Here's how the part is built. I have some questions about the finished solid (model axes, mm). Face numbers are marked on the shaded views. A direction names the side the tool comes from. Give positions to 0.01 mm unless a question says otherwise; leave off trailing zeros. Write each loop counter-clockwise with the first axis right and the second up, starting at its lowest first coordinate (ties: lowest second). Pieces come first, ordered by that corner, then holes. Notation, with made-up numbers: (59, -4) -> (94, -4) arc R15 ccw to (94, 0) -> close; hole circle Ø2 at (40.5, 33.25). An arc over 180 degrees is marked (long way). Return JSON: item names as keys, results as strings.
from build123d import *

# Parameters (mm, degrees)
SKETCH_1_W      = 25.1
SKETCH_1_H      = 19
EXTRUDE_1_DEPTH = 0.8
SKETCH_2_W      = 12.4
SKETCH_2_H      = 17
EXTRUDE_2_DEPTH = 3.75
EXTRUDE_3_DEPTH = 0.1


with BuildPart() as part:
    # Эскиз1 → Бобышка-Вытянуть1 (new body)
    with BuildSketch(Plane.XY):
        Rectangle(SKETCH_1_W, SKETCH_1_H)
    extrude(amount=EXTRUDE_1_DEPTH)

    # Эскиз2 → Бобышка-Вытянуть2 (add)
    with BuildSketch(Plane.XY.offset(0.8)):
        with Locations((-6.35, 0)):
            Rectangle(SKETCH_2_W, SKETCH_2_H)
        with Locations((6.35, 0)):
            Rectangle(SKETCH_2_W, SKETCH_2_H)
    extrude(amount=EXTRUDE_2_DEPTH)

    # Эскиз3 → Бобышка-Вытянуть3 (add)
    with BuildSketch(Plane.XY.offset(4.55)):
        Polygon((-2.02468415, 6.47520488), (-2.557441739, 7.110113629), (-7.634747282, 7.110113629), (-8.413649878, 6.456542649), (-7.703502871, 5.610259577), (-3.055232199, 5.610259577), align=None)
        Polygon((-1.29882158, 5.610259577), (-2.115441527, 0.979668914), (-3.03146241, 0.211374323), (-3.644937808, 0.942733655), (-2.862323662, 5.380419467), (-1.831775613, 6.245561214), align=None)
        Polygon((-7.933342981, 5.41735104), (-8.715781578, 0.979668914), (-9.631802461, 0.211374323), (-10.245102311, 0.942933785), (-9.422392583, 5.610259577), (-8.643686432, 6.263830557), align=None)
        Polygon((-8.523069486, 0.750025248), (-3.874798814, 0.750025248), (-3.260537626, 0), (-4.176367833, -0.749828804), (-8.824808297, -0.749828804), (-9.438886615, 0), align=None)
        Polygon((-3.984111693, -0.979995723), (-3.06780465, -0.211374323), (-2.454394697, -0.942560314), (-3.277521077, -5.609847275), (-4.056117123, -6.263437667), (-4.766565605, -5.416832984), align=None)
        Polygon((-9.054648407, -0.942737341), (-9.668341145, -0.211177879), (-10.584362029, -0.979472469), (-11.400981975, -5.609866688), (-10.868224387, -6.244775436), (-9.837186085, -5.37955138), align=None)
        Polygon((-4.996497129, -5.609866688), (-9.644374912, -5.609866688), (-10.674989606, -6.475066276), (-10.142165372, -7.110113629), (-5.064859829, -7.110113629), (-4.286153678, -6.456346204), align=None)
        Polygon((10.67560373, 6.47520488), (10.142846141, 7.110113629), (5.065540598, 7.110113629), (4.286638002, 6.456542649), (4.996785009, 5.610259577), (9.64505568, 5.610259577), align=None)
        Polygon((11.4014663, 5.610259577), (10.584846353, 0.979668914), (9.66882547, 0.211374323), (9.055350072, 0.942733655), (9.837964217, 5.380419467), (10.868512267, 6.245561214), align=None)
        Polygon((4.766944899, 5.41735104), (3.984506302, 0.979668914), (3.068485419, 0.211374323), (2.455185569, 0.942933785), (3.277895297, 5.610259577), (4.056601448, 6.263830557), align=None)
        Polygon((4.177218394, 0.750025248), (8.825489066, 0.750025248), (9.439750254, 0), (8.523920047, -0.749828804), (3.875479583, -0.749828804), (3.261401265, 0), align=None)
        Polygon((8.716176187, -0.979995723), (9.63248323, -0.211374323), (10.245893183, -0.942560314), (9.422766803, -5.609847275), (8.644170756, -6.263437667), (7.933722275, -5.416832984), align=None)
        Polygon((3.645639473, -0.942737341), (3.031946734, -0.211177879), (2.115925851, -0.979472469), (1.299305904, -5.609866688), (1.832063493, -6.244775436), (2.863101795, -5.37955138), align=None)
        Polygon((7.70379075, -5.609866688), (3.055912968, -5.609866688), (2.025298274, -6.475066276), (2.558122507, -7.110113629), (7.635428051, -7.110113629), (8.414134202, -6.456346204), align=None)
    extrude(amount=EXTRUDE_3_DEPTH)


solid = part.part
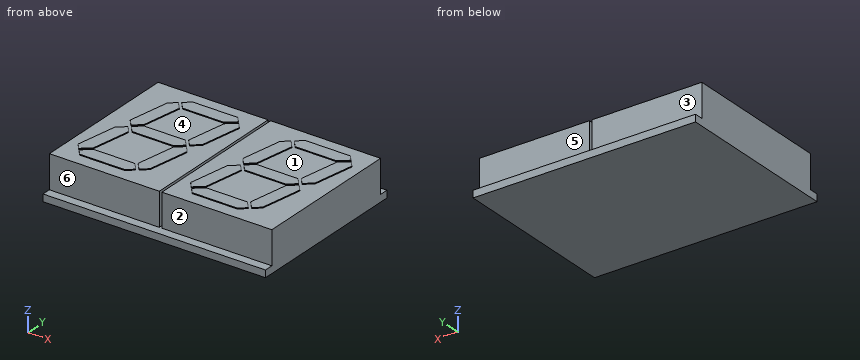
1. If I drill on line 1 (X direction, y = -7.5, z = 4.25); line 2 (Y direction, x = 2.75, z = 3.55); line 3 (Z direction, x = -4.75, y = -3.25), over which ranges is the centre line in solid material (lowest first)? Write a range as [from, to].
Taken from the geometry:
{"line 1": "x = [-12.55, -0.15], [0.15, 12.55]", "line 2": "y = [-8.5, 8.5]", "line 3": "z = [0, 4.55]"}
2. Suppose I cut it at A-A, the plane x = 1. List the corners of the cut face in (y, z) for me, and give its area (4 significant figures).
Taken from the geometry:
{"outline": "(-9.5, 0) -> (9.5, 0) -> (9.5, 0.8) -> (8.5, 0.8) -> (8.5, 4.55) -> (-8.5, 4.55) -> (-8.5, 0.8) -> (-9.5, 0.8) -> close", "area": "78.95 mm²"}
3. If we mould it in two halves opening along Y, with no side actions, what happens to the marked faces 1, 2 and 3? For each: released by +Y, released by -Y, zero draft, split by the parting line, or undercut.
Taken from the geometry:
{"face 1": "undercut", "face 2": "released by -Y", "face 3": "released by +Y"}
4. Suppose I cut it at D-D, the plane y = 4. List the corners of the cut face in (x, z) for me.
Taken from the geometry:
{"outline": "(-12.55, 0) -> (12.55, 0) -> (12.55, 4.55) -> (11.12, 4.55) -> (11.12, 4.65) -> (9.59, 4.65) -> (9.59, 4.55) -> (4.52, 4.55) -> (4.52, 4.65) -> (2.99, 4.65) -> (2.99, 4.55) -> (0.15, 4.55) -> (0.15, 0.8) -> (-0.15, 0.8) -> (-0.15, 4.55) -> (-1.58, 4.55) -> (-1.58, 4.65) -> (-3.11, 4.65) -> (-3.11, 4.55) -> (-8.18, 4.55) -> (-8.18, 4.65) -> (-9.71, 4.65) -> (-9.71, 4.55) -> (-12.55, 4.55) -> close"}
5. Suppose I cut it at C-C, the plane y = 7.75. List the corners of the cut face in (x, z) for me, and give its area (3 significant figures).
Taken from the geometry:
{"outline": "(-12.55, 0) -> (12.55, 0) -> (12.55, 4.55) -> (0.15, 4.55) -> (0.15, 0.8) -> (-0.15, 0.8) -> (-0.15, 4.55) -> (-12.55, 4.55) -> close", "area": "113 mm²"}
6. For pin 1 Ø1.1 at (x, z) = (4, 3) entering from +Y; pin 2 Ø1.5 at (x, y) = (-2, -4) entering from +Z; pin 3 Ø1.9 at (x, z) = (4.5, 3.5) entering from -Y, each with a flat end and sliding along its axis, tell me the tip position at first contact or that it passes through.
Taken from the geometry:
{"pin 1": "stops at y = 8.5", "pin 2": "stops at z = 4.55", "pin 3": "stops at y = -8.5"}
7. Suppose I cut it at B-B, the plane z = 2.95. List the corners of the cut face in (x, y) for me, and give its area (3 significant figures).
Taken from the geometry:
{"outline": "(-12.55, -8.5) -> (-0.15, -8.5) -> (-0.15, 8.5) -> (-12.55, 8.5) -> close; (0.15, -8.5) -> (12.55, -8.5) -> (12.55, 8.5) -> (0.15, 8.5) -> close", "area": "422 mm²"}
8. Which directions (+Z, -Z, +X, -X, +Y, -Y) give clear straight access to the entire face, cutting with the end or side of a thin tool? Please do the marked faces 4, 5 and 6.
Taken from the geometry:
{"face 4": "+Z", "face 5": "+Z, +X, -X, +Y", "face 6": "+Z, +X, -X, -Y"}
